Geometry check sheet. Reference: the model listing, model coordinates, mm. Face numbers are marked on the shaded views. A direction names the side the tool comes from. Round coordinates to 2 decimals unless told otherwise and drop trailing zeros. Order: outer loops, then holes, each group sorted by start corner. A loop starts at its lowest first (then second) coordinate and runs counter-clockwise, first axis right, second up. Notation, with made-up numbers: (60, 63) - (116, 63) arc R10 cw to (116, 74) - close; hole circle Ø4 at (-36.5, -17). An arc over 180 degrees is marked (long way). Use a Markdown table: item, result. Add a question column.
(1) Section check C-C on z = 17.75. Record the boundary of the cut face in (x, y), then the cut area to 3 significant figures.
(2) Thickness scan on line 1 along X through (y, z) = (-6.25, 10.25); line 2 along X through (y, z) = (-6.5, 11.75); line 3 along X through (y, z) = (-3.5, 16.5). Record the ranges inside material, lowest first. Write a range as [from, to].
(3) Section check D-D on x = -38. Record the boundary of the cut face in (y, z).
(4) Mould release check, pull along X, two halves, no side actions. Record for the marked faces 3, 4 and 5: released by +X, released by -X, zero draft, split by the parting line, or undercut.
(5) Section check B-B on y = -1. Record the boundary of the cut face in (x, z), then the cut area to 3 significant figures.
(6) Access from +Z, -Z, +X, -X, +Y, -Y to the whole of each face (thin tool, end or side, straight path). Record for the marked faces 1 and 2.
(7) Gauge pin test, flat ends, axial feed: P1, Ø8, axis at x = -12.19, z = 10.21, coming from the -Y side; P2, Ø6, axis at x = -36.5, z = 9.5, coming from the +Y side. Record the tip position at first contact, or that the pin passes through.
(8) Section check A-A on y = -3.25. Record the boundary of the cut face in (x, z).
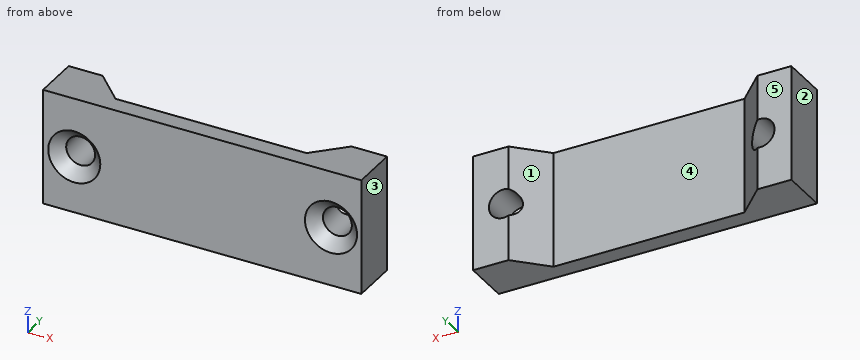
```python
from build123d import *

# Parameters (mm, degrees)
F0_W        = 55
F0_H        = 8
F1_DEPTH    = 20
F2_R        = 2.5
F3_DEPTH    = 35.3
F4_W        = 33
F4_H        = 86
F5_DEPTH    = 5
F6_SIZE     = 2
F7_SIZE     = 2
F8_T4_DEPTH = 45.7168298797
F8_T9_DEPTH = 45.7168298797


# Not quite as in the source:
# - a fillet or chamfer that OpenCascade refuses, or shapes differently, is made with other operations: its cross-section is extruded or revolved along the edge and cut away or added


with BuildPart() as f1:
    # F0 (on Top) → F1 (new body)
    with BuildSketch(Plane.XY):
        with Locations((-34.4500018656, -4)):
            Rectangle(F0_W, F0_H)
    extrude(amount=F1_DEPTH)

    # F2 (on Front) → F3 (cut)
    with BuildSketch(Plane.XZ):
        with Locations((-56.5492250025, 9.7595239058)):
            Circle(F2_R)
        with Locations((-12.1940001845, 10.2066537365)):
            Circle(F2_R)
    extrude(amount=F3_DEPTH, mode=Mode.SUBTRACT)

    # F4 (on Front) → F5 (cut)
    with BuildSketch(Plane.XZ):
        with Locations((-34.5833339691, 26.0833319575)):
            Rectangle(F4_W, F4_H)
    extrude(amount=F5_DEPTH, mode=Mode.SUBTRACT)

    # F6
    f6_edges = [f1.edges().sort_by_distance(p)[0] for p in [
        (-14.694, -8, 10.206654),
    ]]
    chamfer(f6_edges, length=F6_SIZE)

    # F7
    f7_edges = [f1.edges().sort_by_distance(p)[0] for p in [
        (-59.049225, -8, 9.759524),
    ]]
    chamfer(f7_edges, length=F7_SIZE)

    # F8: chamfer of 5 on 2 edges, made by hand


with BuildPart() as f8_tool2:
    # F8_s3 → F8_t4 (new body)
    with BuildSketch(Plane.XY.offset(32.8584149398)):
        Polygon((-56.0833339691, 0), (-51.0833339691, -5), (-51.0833339691, 0), align=None)
    extrude(amount=-F8_T4_DEPTH)

    split(bisect_by=Plane.XZ.offset(5), keep=Keep.BOTTOM)


with BuildPart() as f1_1:
    add(f1.part)

    # F8_t1: cut F8_tool2
    add(f8_tool2.part, mode=Mode.SUBTRACT)


with BuildPart() as f8_tool7:
    # F8_s8 → F8_t9 (new body)
    with BuildSketch(Plane.XY.offset(-12.8584149398)):
        Polygon((-18.0833339691, -5), (-13.0833339691, 0), (-18.0833339691, 0), align=None)
    extrude(amount=F8_T9_DEPTH)

    split(bisect_by=Plane.XZ.offset(5), keep=Keep.BOTTOM)


with BuildPart() as f1_2:
    add(f1_1.part)

    # F8_t6: cut F8_tool7
    add(f8_tool7.part, mode=Mode.SUBTRACT)


solid = f1_2.part
```
Check sheet entries:
| question | item | result |
|---|---|---|
| 1 | outline | (-61.95, -8) - (-6.95, -8) - (-6.95, 0) - (-13.08, 0) - (-18.08, -5) - (-51.08, -5) - (-56.08, 0) - (-61.95, 0) - close |
| 1 | area | 250 mm2 |
| 2 | line 1 | x = [-61.95, -59.26], [-53.84, -14.94], [-9.44, -6.95] |
| 2 | line 2 | x = [-61.95, -58.79], [-54.3, -14.77], [-9.62, -6.95] |
| 2 | line 3 | x = [-61.95, -52.58], [-16.58, -6.95] |
| 3 | outline | (-8, 0) - (-5, 0) - (-5, 20) - (-8, 20) - close |
| 4 | face 3 | released by +X |
| 4 | face 4 | undercut |
| 4 | face 5 | zero draft |
| 5 | outline | (-61.95, 0) - (-55.08, 0) - (-55.08, 7.73) arc R2.5 cw (long way) to (-55.08, 11.78) - (-55.08, 20) - (-61.95, 20) - close; (-14.08, 0) - (-6.95, 0) - (-6.95, 20) - (-14.08, 20) - (-14.08, 11.84) arc R2.5 cw (long way) to (-14.08, 8.57) - close |
| 5 | area | 245 mm2 |
| 6 | face 1 | +Z, -Z, +Y |
| 6 | face 2 | +Z, -Z, -X, +Y, -Y |
| 7 | P1 | stops at y = -7.51 |
| 7 | P2 | stops at y = -5 |
| 8 | outline | (-61.95, 0) - (-52.83, 0) - (-52.83, 20) - (-61.95, 20) - close; (-16.33, 0) - (-6.95, 0) - (-6.95, 20) - (-16.33, 20) - close; hole circle Ø5 at (-56.55, 9.76); hole circle Ø5 at (-12.19, 10.21) |
